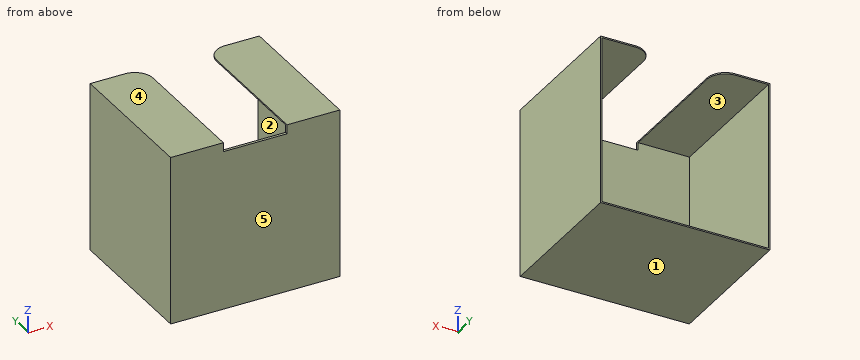
```python
from build123d import *

# Parameters (mm, degrees)
SKETCH2_W           = 93
SKETCH2_H           = 93
BOSS_EXTRUDE2_DEPTH = 80
SKETCH3_W           = 91.5
SKETCH3_H           = 91.5
CUT_EXTRUDE1_DEPTH  = 78.5
SKETCH6_W           = 35
SKETCH6_H           = 80
CUT_EXTRUDE2_DEPTH  = 5
FILLET1_R           = 10
FILLET2_R           = 10


with BuildPart() as part:
    # Sketch2 → Boss-Extrude2 (new body)
    with BuildSketch(Plane(origin=(0, 0, 0), x_dir=(1, 0, 0), z_dir=(0, 1, 0))):
        Rectangle(SKETCH2_W, SKETCH2_H)
    extrude(amount=BOSS_EXTRUDE2_DEPTH)

    # Sketch3 → Cut-Extrude1 (cut)
    with BuildSketch(Plane(origin=(0, 80, 0), x_dir=(1, 0, 0), z_dir=(0, 1, 0))):
        Rectangle(SKETCH3_W, SKETCH3_H)
    extrude(amount=-CUT_EXTRUDE1_DEPTH, mode=Mode.SUBTRACT)

    # Sketch6 → Cut-Extrude2 (cut)
    with BuildSketch(Plane.XY.offset(46.5)):
        with Locations((0, 40)):
            Rectangle(SKETCH6_W, SKETCH6_H)
    extrude(amount=-CUT_EXTRUDE2_DEPTH, mode=Mode.SUBTRACT)

    # Fillet1
    fillet1_edges = [part.edges().sort_by_distance(p)[0] for p in [
        (-17.5, 80, 46.125),
    ]]
    fillet(fillet1_edges, radius=FILLET1_R)

    # Fillet2
    fillet2_edges = [part.edges().sort_by_distance(p)[0] for p in [
        (17.5, 80, 46.125),
    ]]
    fillet(fillet2_edges, radius=FILLET2_R)


solid = part.part
```
Build history of the part. All positions in model axes, mm. Face numbers are marked on the shaded views. A direction names the side the tool comes from. Round coordinates to 2 decimals unless told otherwise and drop trailing zeros. Write each loop counter-clockwise with the first axis right and the second up, starting at its lowest first coordinate (ties: lowest second). Pieces come first, ordered by that corner, then holes.
1) 3-axis set-ups, long thin cutter, end or side, ignore diameter. For the marked faces 1 and 2: which of +Z, -Z, +X, -X, +Y, -Y reach the whole face in a straight line?
2) Mould opens along Z. For the marked faces 3, 4 and 5 say: +Z half, -Z half, draft (parallel to the pull), parting line (faces both ways), or undercut.
3) Band-saw the part on D-D, the plane x = 10. List the corners of the cut face in (y, z), and give its area (3 significant figures).
4) Pin check, flat tips, straight feed: pin 1 (5 mm diameter, centred on x = 22.5, z = 24.5, fed in from +Y); pin 2 (1.6 mm diameter, centred on x = 7, y = 1, fed in from +Z); pin 3 (8 mm diameter, centred on x = 7.5, y = 24.5, fed in from +Z). Stop position of each tip, or through.
5) Band-saw the part on C-C, the plane x = -24. List the corners of the cut face in (y, z), and give its area (3 significant figures).
6) Drill centre lines: probe 1 along X at (y, z) = (67, 14); probe 2 along Z at (x, y) = (-17, 69). Where is each one in solid material? Low to high.
7) Band-saw the part on B-B, the plane y = 44. List the corners of the cut face in (x, z), and give its area (4 significant figures).
8) Band-saw the part on A-A, the plane z = 17.5. List the corners of the cut face in (x, y), and give its area (3 significant figures).
Ans:
1. face 1: -Z, +X, -X, +Y, -Y
1. face 2: +Y
2. face 3: undercut
2. face 4: +Z half
2. face 5: draft
3. outline: (0, -46.5) - (80, -46.5) - (80, -45.75) - (1.5, -45.75) - (1.5, 41.5) - (0, 41.5) - close
3. area: 191 mm2
4. pin 1: stops at y = 1.5
4. pin 2: stops at z = 41.5
4. pin 3: stops at z = -45.75
5. outline: (0, -46.5) - (80, -46.5) - (80, -45.75) - (1.5, -45.75) - (1.5, 45.75) - (79.37, 45.75) - (79.37, 46.5) - (0, 46.5) - close
5. area: 257 mm2
6. probe 1: x = -46.5 to -45.75, 45.75 to 46.5
6. probe 2: z = -46.5 to -45.75
7. outline: (-46.5, -46.5) - (46.5, -46.5) - (46.5, 46.5) - (17.5, 46.5) - (17.5, 45.75) - (45.75, 45.75) - (45.75, -45.75) - (-45.75, -45.75) - (-45.75, 45.75) - (-17.5, 45.75) - (-17.5, 46.5) - (-46.5, 46.5) - close
7. area: 250.5 mm2
8. outline: (-46.5, 0) - (46.5, 0) - (46.5, 80) - (45.75, 80) - (45.75, 1.5) - (-45.75, 1.5) - (-45.75, 80) - (-46.5, 80) - close
8. area: 257 mm2
